Check sheet for the modelled part. Datum: model origin and axes. Units: mm. A direction names the side the tool comes from. Coordinates: 2 decimals unless noted, no trailing zeros. Loops run counter-clockwise (first coordinate to the right, second up) from the corner with the lowest first, then second, coordinate; pieces in that order, holes last.
from build123d import *

# Parameters (mm, degrees)
ESQUISSE1_R                  = 9.125
ESQUISSE1_R_2                = 6.125
BOSS_EXTRU_1_DEPTH           = 25
ESQUISSE13_W                 = 33.25
ESQUISSE13_H                 = 25
BOSS_EXTRU_10_DEPTH          = 3
BOSS_EXTRU_11_DEPTH          = 3
BOSS_EXTRU_11_DEPTH_BACK     = 1.503194454
ESQUISSE14_W                 = 16.5
ESQUISSE14_H                 = 25
ENL_V_MAT_EXTRU_1_DEPTH      = 38.311344137
ENL_V_MAT_EXTRU_1_DEPTH_BACK = 38.311344137
ESQUISSE15_R                 = 1.5
CONG_1_R                     = 10


with BuildPart() as part:
    # Esquisse1 → Boss.-Extru.1 (new body)
    # profile 1 of 2: a face of its own
    with BuildSketch(Plane.XY):
        Circle(ESQUISSE1_R)
        Circle(ESQUISSE1_R_2, mode=Mode.SUBTRACT)
    # profile 2 of 2: a face of its own
    with BuildSketch(Plane.XY):
        with BuildLine():
            ThreePointArc((9.125, 0), (0, -9.125), (-9.125, 0))
            Line((-9.125, 0), (-9.125, -10.60590961))
            Line((-9.125, -10.60590961), (9.125, -10.60590961))
            Line((9.125, -10.60590961), (9.125, 0))
        make_face()
    extrude(amount=BOSS_EXTRU_1_DEPTH)

    # Esquisse13 → Boss.-Extru.10 (add)
    with BuildSketch(Plane.XZ.offset(10.60590961)):
        with Locations((-7.5, 12.5)):
            Rectangle(ESQUISSE13_W, ESQUISSE13_H)
    extrude(amount=-BOSS_EXTRU_10_DEPTH)

    # Esquisse14 → Boss.-Extru.11 (add, two sides: drawn at the far end of the back side and taken through both)
    with BuildSketch(Plane(origin=(0, 0, 0), x_dir=(1, 0, 0), z_dir=(0, 1, 0)).offset(-BOSS_EXTRU_11_DEPTH_BACK)):
        with Locations((-15.875, -12.5)):
            Rectangle(ESQUISSE14_W, ESQUISSE14_H)
    extrude(amount=BOSS_EXTRU_11_DEPTH + BOSS_EXTRU_11_DEPTH_BACK)

    # Esquisse15 → Enlèv. mat.-Extru.1 (cut, two sides: drawn at the far end of the back side and taken through both)
    with BuildSketch(Plane(origin=(0, 3, 0), x_dir=(1, 0, 0), z_dir=(0, 1, 0)).offset(-ENL_V_MAT_EXTRU_1_DEPTH_BACK)):
        with Locations(Location((-16.37, -8.333333333, 0), (0, 0, 270))):
            Circle(ESQUISSE15_R)
        with Locations(Location((-16.37, -16.666666667, 0), (0, 0, 270))):
            Circle(ESQUISSE15_R)
    extrude(amount=ENL_V_MAT_EXTRU_1_DEPTH + ENL_V_MAT_EXTRU_1_DEPTH_BACK, mode=Mode.SUBTRACT)

    # Congé1
    cong_1_edges = [part.edges().sort_by_distance(p)[0] for p in [
        (-24.125, -9.10590961, 25),
        (-24.125, 0.748402773, 25),
    ]]
    fillet(cong_1_edges, radius=CONG_1_R)


solid = part.part
(1) Set-up check for faces 4 (the face through (-17, -1.503, 12)), 5 (the face through (-16, 3, 12)), 6 (the face through (-15.919, 0.717, 18.097)): record each of +Z, -Z, +X, -X, +Y, -Y from which the full face is reachable in a straight line by a thin tool's end or side.
(2) Section check B-B, the plane z = 15.75. Enter the section's corners in (x, y) (3 decimals), plus the area to 3 significant figures.
(3) Section check D-D, the plane y = 1.75. Enter the section's corners in (x, z) (3 decimals).
(4) Section check C-C, the plane y = -8.25. Enter the section's corners in (x, z) (3 decimals), plus the area to 3 significant figures.
(5) Scan lines: line 1 along Z through (x, y) = (-16.37, 0.15); line 2 along Y through (x, z) = (0, 17.75) (3 decimals); line 3 along X through (y, z) = (0.25, 11.5) (3 decimals). Record each from-to range of solid material in increasing order.
(6) Draft check along Z on faces 1 (the face through (-21.118, -9.085, 22.148)), 2 (the face through (-17.7, 0.72, 9.03)), 3 (the face through (-9.125, -5, 12)). Enter one of: pulls with the +Z half, pulls with the -Z half, needs draft (parallel to the pull), parting line crosses it, or undercut.
(7) Gauge pin test, flat ends, axial feed: P1, Ø2, axis at y = 6.5, z = 6.5, coming from the -X side; P2, Ø12.5, axis at x = -14, z = 9, coming from the +Y side; P3, Ø2, axis at x = 3, y = 7, coming from the -Z side; P4, Ø12, axis at x = -9.5, z = 3, coming from the +Y side. Record the tip position at first contact, or that the pin passes through.
(8) Section check A-A, the plane x = 0. Enter the section's corners in (y, z) (3 decimals).
Determined:
1. face 4: +Z, -Z, -X
1. face 5: +Z, -Z, -X, +Y
1. face 6: +Y, -Y
2. outline: (-24.097, -10.606) - (-17.557, -10.606) - (-17.557, -7.606) - (-24.097, -7.606) - close; (-24.097, -1.503) - (-17.557, -1.503) - (-17.557, 3) - (-24.097, 3) - close; (-15.183, -10.606) - (9.125, -10.606) - (9.125, 0) arc R9.125 ccw to (-8.618, 3) - (-15.183, 3) - (-15.183, -1.503) - (-9.125, -1.503) - (-9.125, -7.606) - (-15.183, -7.606) - close; hole circle Ø12.25 at (0, 0)
2. area: 302 mm2
3. outline: (-24.125, 0) - (-5.87, 0) - (-5.87, 25) - (-14.125, 25) arc R10 ccw to (-24.125, 15) - close; (5.87, 0) - (8.956, 0) - (8.956, 25) - (5.87, 25) - close; hole circle Ø3 at (-16.37, 8.333); hole circle Ø3 at (-16.37, 16.667)
4. outline: (-24.125, 0) - (9.125, 0) - (9.125, 25) - (-14.125, 25) arc R10 ccw to (-24.125, 15) - close; hole circle Ø3 at (-16.37, 8.333); hole circle Ø3 at (-16.37, 16.667)
4. area: 796 mm2
5. line 1: z = 0 to 6.83, 9.83 to 15.17, 18.17 to 24.74
5. line 2: y = -10.606 to -6.125, 6.125 to 9.125
5. line 3: x = -24.125 to -6.12, 6.12 to 9.122
6. face 1: pulls with the +Z half
6. face 2: undercut
6. face 3: needs draft
7. P1: stops at x = -7.28
7. P2: stops at y = 4.82
7. P3: stops at z = 0
7. P4: stops at y = 8.43
8. outline: (-10.606, 0) - (-6.125, 0) - (-6.125, 25) - (-10.606, 25) - close; (6.125, 0) - (9.125, 0) - (9.125, 25) - (6.125, 25) - close
